```python
from build123d import *

# Parameters (mm, degrees)
ESBO_O10_W               = 11.5
ESBO_O10_H               = 11.5
ESBO_O10_R               = 2.5
RESSALTO_EXTRUS_O4_DEPTH = 8
CHANFRO2_SIZE            = 3.5
ESBO_O12_R               = 1.925
CORTE_EXTRUS_O4_DEPTH    = 3
ESBO_O17_R               = 1.925
CORTE_EXTRUS_O5_DEPTH    = 3
RESSALTO_EXTRUS_O5_START = -4.2
ESBO_O18_R               = 2.5
ESBO_O18_R_2             = 2.25
RESSALTO_EXTRUS_O5_DEPTH = 4.2
ESBO_O19_R               = 1.625
CORTE_EXTRUS_O6_DEPTH    = 14.431064984
ESBO_O20_R               = 1.625
CORTE_EXTRUS_O7_DEPTH    = 14.431065043
RESSALTO_EXTRUS_O6_START = -3.4
ESBO_O24_W               = 24
ESBO_O24_H               = 11.5
ESBO_O24_R               = 2.25
RESSALTO_EXTRUS_O6_DEPTH = 3.4
CORTE_EXTRUS_O8_DEPTH    = 3
ESBO_O26_R               = 1.9
CORTE_EXTRUS_O9_DEPTH    = 16.323919261
CORTE_EXTRUS_O10_DEPTH   = 15.079151286
FILETE3_R                = 1
FILETE4_R                = 0.5
ESBO_O30_R               = 4.5
CORTE_EXTRUS_O11_DEPTH   = 1.2


with BuildPart() as part:
    # Esboço10 → Ressalto-extrusão4 (new body)
    with BuildSketch(Plane(origin=(0, 0, 0), x_dir=(1, 0, 0), z_dir=(0, 1, 0))):
        Rectangle(ESBO_O10_W, ESBO_O10_H)
        with Locations(Location((0, 0, 0), (0, 0, 270))):
            Circle(ESBO_O10_R, mode=Mode.SUBTRACT)
    extrude(amount=RESSALTO_EXTRUS_O4_DEPTH)

    # Chanfro2
    chanfro2_edges = [part.edges().sort_by_distance(p)[0] for p in [
        (5.75, 4, 5.75),
        (-5.75, 4, 5.75),
        (-5.75, 4, -5.75),
        (5.75, 4, -5.75),
    ]]
    chamfer(chanfro2_edges, length=CHANFRO2_SIZE)

    # Esboço12 → Corte-extrusão4 (cut)
    with BuildSketch(Plane(origin=(-4, 0, 4), x_dir=(0.7071067811865465, 0, 0.7071067811865487), z_dir=(-0.7071067811865487, 0, 0.7071067811865465))):
        with Locations((0, 2.3)):
            Circle(ESBO_O12_R)
    corte_extrus_o4 = extrude(amount=-CORTE_EXTRUS_O4_DEPTH, mode=Mode.SUBTRACT)

    # Esboço17 → Corte-extrusão5 (cut)
    with BuildSketch(Plane(origin=(4, 0, 4), x_dir=(0.7071067811865489, 0, -0.7071067811865462), z_dir=(0.7071067811865462, 0, 0.7071067811865489))):
        with Locations((0, 2.3)):
            Circle(ESBO_O17_R)
    corte_extrus_o5 = extrude(amount=-CORTE_EXTRUS_O5_DEPTH, mode=Mode.SUBTRACT)

    # Espelhar1: Corte-extrusão4 across plane
    add(corte_extrus_o4.mirror(Plane.XY), mode=Mode.SUBTRACT)

    # Espelhar2: Corte-extrusão5 across plane
    add(corte_extrus_o5.mirror(Plane.XY), mode=Mode.SUBTRACT)

    # Esboço18 → Ressalto-extrusão5 (add)
    with BuildSketch(Plane(origin=(0, 8, 0), x_dir=(1, 0, 0), z_dir=(0, 1, 0)).offset(RESSALTO_EXTRUS_O5_START)):
        with Locations(Location((0, 0, 0), (0, 0, 270))):
            Circle(ESBO_O18_R)
        with Locations(Location((0, 0, 0), (0, 0, 270))):
            Circle(ESBO_O18_R_2, mode=Mode.SUBTRACT)
    extrude(amount=RESSALTO_EXTRUS_O5_DEPTH)

    # Esboço19 → Corte-extrusão6 (cut, through all)
    with BuildSketch(Plane(origin=(-1.878679656, 0, 1.878679656), x_dir=(0.7071067811865465, 0, 0.7071067811865486), z_dir=(-0.7071067811865486, 0, 0.7071067811865465))):
        with Locations(Location((0, 2.3, 0), (0, 0, 67.380135052))):
            Circle(ESBO_O19_R)
    extrude(amount=-CORTE_EXTRUS_O6_DEPTH, mode=Mode.SUBTRACT)

    # Esboço20 → Corte-extrusão7 (cut, through all)
    with BuildSketch(Plane(origin=(1.878679656, 0, 1.878679656), x_dir=(0.7071067811865488, 0, -0.7071067811865464), z_dir=(0.7071067811865464, 0, 0.7071067811865488))):
        with Locations((0, 2.3)):
            Circle(ESBO_O20_R)
    extrude(amount=-CORTE_EXTRUS_O7_DEPTH, mode=Mode.SUBTRACT)

    # Esboço24 → Ressalto-extrusão6 (add)
    with BuildSketch(Plane(origin=(0, 8, 0), x_dir=(1, 0, 0), z_dir=(0, 1, 0)).offset(RESSALTO_EXTRUS_O6_START)):
        Rectangle(ESBO_O24_W, ESBO_O24_H)
        with Locations(Location((0, 0, 0), (0, 0, 270))):
            Circle(ESBO_O24_R, mode=Mode.SUBTRACT)
    extrude(amount=RESSALTO_EXTRUS_O6_DEPTH)

    # Esboço25 → Corte-extrusão8 (cut)
    with BuildSketch(Plane.XZ.offset(-4.6)):
        Polygon((-8.75, 3.059956427), (-11.4, 1.529978213), (-11.4, -1.529978213), (-8.75, -3.059956427), (-6.1, -1.529978213), (-6.1, 1.529978213), align=None)
        Polygon((6.1, 1.529978213), (8.75, 3.059956427), (11.4, 1.529978213), (11.4, -1.529978213), (8.75, -3.059956427), (6.1, -1.529978213), align=None)
    extrude(amount=-CORTE_EXTRUS_O8_DEPTH, mode=Mode.SUBTRACT)

    # Esboço26 → Corte-extrusão9 (cut, through all)
    with BuildSketch(Plane.XZ.offset(-7.6)):
        with Locations(Location((-8.75, 0, 0), (0, 0, 270))):
            Circle(ESBO_O26_R)
        with Locations(Location((8.75, 0, 0), (0, 0, 90))):
            Circle(ESBO_O26_R)
    extrude(amount=-CORTE_EXTRUS_O9_DEPTH, mode=Mode.SUBTRACT)

    # Esboço27 → Corte-extrusão10 (cut, through all)
    with BuildSketch(Plane.XZ.offset(-4.6)):
        Polygon((-12, 5.75), (-12, 2.25), (-5.937822174, 5.75), align=None)
        Polygon((-5.937822174, -5.75), (-12, -5.75), (-12, -2.25), align=None)
        Polygon((12, -5.75), (12, -2.25), (5.937822174, -5.75), align=None)
        Polygon((5.937822174, 5.75), (12, 5.75), (12, 2.25), align=None)
    extrude(amount=-CORTE_EXTRUS_O10_DEPTH, mode=Mode.SUBTRACT)

    # Filete3
    filete3_edges = [part.edges().sort_by_distance(p)[0] for p in [
        (12, 6.3, 2.25),
        (5.937822174, 6.3, 5.75),
        (5.937822174, 6.3, -5.75),
        (12, 6.3, -2.25),
        (-12, 6.3, -2.25),
        (-5.937822174, 6.3, -5.75),
        (-5.937822174, 6.3, 5.75),
        (-12, 6.3, 2.25),
    ]]
    fillet(filete3_edges, radius=FILETE3_R)

    # Filete4
    filete4_edges = [part.edges().sort_by_distance(p)[0] for p in [
        (-2.25, 2.3, 5.75),
        (-5.75, 2.3, -2.25),
        (5.75, 2.3, 2.25),
        (2.25, 2.3, -5.75),
        (-2.25, 2.3, -5.75),
        (5.75, 2.3, -2.25),
        (2.25, 2.3, 5.75),
        (-5.75, 2.3, 2.25),
    ]]
    fillet(filete4_edges, radius=FILETE4_R)

    # Esboço30 → Corte-extrusão11 (cut)
    with BuildSketch(Plane(origin=(0, 8, 0), x_dir=(1, 0, 0), z_dir=(0, 1, 0))):
        with Locations(Location((0, 0, 0), (0, 0, 270))):
            Circle(ESBO_O30_R)
    extrude(amount=-CORTE_EXTRUS_O11_DEPTH, mode=Mode.SUBTRACT)


solid = part.part
```
Input: part model. Units: mm. Frame: model coordinates. A direction names the side the tool comes from. Round coordinates to 2 decimals unless told otherwise and drop trailing zeros. Order: outer loops, then holes, each group sorted by start corner. A loop starts at its lowest first (then second) coordinate and runs counter-clockwise, first axis right, second up. Notation, with made-up numbers: (16, 42) - (50, 42) arc R16 cw to (50, 67) - close; hole circle Ø11 at (60, 19). An arc over 180 degrees is marked (long way). One line per question, with ' | ' between items. Start each with the question number.
1) Cut plane B-B, the plane x = 8.5. Return the cut outline in (y, z), then the cut area to 3 significant figures.
2) Pull-direction query (Z, two-part tool) for faces 1 (the cylindrical face through (0.676, 5.279, 2.146)), 2 (the flat face through (-3, 8, -4)), 3 (the cylindrical face through (11.87, 6.324, 2.166)); classes: +Z half, -Z half, draft (parallel to the pull), parting line (faces both ways), or undercut.
3) Set-up query: faces 4 (the cylindrical face through (-3.25, 0.42, -2.66)), 5 (the flat face through (5.75, 2, 0)), 6 (the cylindrical face through (1.352, 7.408, 4.292)), 7 (the flat face through (5.9, 4.6, -0.5)), 8 (the flat face through (-7.406, 6.079, 2.284)). Return all of +Z, -Z, +X, -X, +Y, -Y with unobstructed straight access to the full face (end or side cutting, diameter ignored); none if empty.
4) Ray query, probe 1 along X at (y, z) = (7.9, 0); probe 2 along X at (y, z) = (7.35, 0); probe 3 along X at (y, z) = (5.25, 2.5). Return the intervals inside material, ascending.
5) Contact query for flat-ended pins moving along their axis: P1, Ø0.6, axis at x = -0.5, z = 2, coming from the -Y side; P2, Ø4, axis at y = 1, z = -1, coming from the -X side; P3, Ø2, axis at y = 2, z = -0.5, coming from the +X side. Output: stop coordinate, or through.
6) Cut plane A-A, the plane y = 5.25. Give the number of separate pieces and of enclosed holes in the cut face, then the cut area to 3 significant figures.
Worked out:
1) outline: (4.6, -4.27) - (8, -4.27) - (8, -1.88) - (7.6, -1.88) - (7.6, -2.92) - (4.6, -2.92) - close; (4.6, 2.92) - (7.6, 2.92) - (7.6, 1.88) - (8, 1.88) - (8, 4.27) - (4.6, 4.27) - close | area: 10.0 mm^2
2) face 1: undercut | face 2: draft | face 3: +Z half
3) face 4: none | face 5: +Z, -Z, +X, -Y | face 6: +Y | face 7: +X, -Y | face 8: -Y
4) probe 1: x = -12 to -10.65, -6.85 to -4.5, 4.5 to 6.85, 10.65 to 12 | probe 2: x = -12 to -11.4, -6.1 to -4.5, 4.5 to 6.1, 11.4 to 12 | probe 3: x = -11.56 to -9.72, -7.78 to 7.78, 9.72 to 11.56
5) P1: stops at y = 3.8 | P2: stops at x = -5.75 | P3: stops at x = 5.75
6) separate pieces: 1 | enclosed holes: 3 | area: 169 mm^2
